Source: CAD feature listing. Evaluate the final solid. Frame: model axes, mm. A direction names the side the tool comes from. Round coordinates to 2 decimals unless told otherwise and drop trailing zeros. Loops run counter-clockwise (first coordinate to the right, second up) from the corner with the lowest first, then second, coordinate; pieces in that order, holes last.
(1) Material intervals for probe 1 along Z at (x, y) = (-35.5, 1.35); probe 2 along X at (y, z) = (0.1, -15); probe 3 along Z at (x, y) = (-11.5, 1.3), sorted ascending.
(2) Section A-A, the plane x = 0. Return the cut outline in (y, z) (3 decimals), plus the area to 3 significant figures.
(3) Section D-D, the plane y = 1.5. Count the separate pieces of the cut face and the enclosed holes in it, plus the area to 3 significant figures.
(4) Section C-C, the plane x = -12.5. Return the cut outline in (y, z), plus the area to 3 significant figures.
(5) Set-up query: faces 1 (the flat face through (1, 0, 1)), 2 (the cylindrical face through (-22.106, 0.986, -21.846)). Return all of +Z, -Z, +X, -X, +Y, -Y with unobstructed straight access to the full face (end or side cutting, diameter ignored); none if empty.
(6) Section B-B, the plane z = 0. Return the cut outline in (x, y), plus the area to 3 significant figures.
(7) First-contact query: pin 1 Ø5 at (x, z) = (35.75, 20.64) entering from +Y; pin 2 Ø1.9 at (x, z) = (0, -41.275) entering from -Y. Flat tips, straight axial feed; report the tip coordinate or a pass-through.
Autodesk Inventor part; units mm, degrees
ref_plane "YZ Plane" through (0, 0, 0) normal (1, 0, 0) x (0, 1, 0)
ref_plane "XZ Plane" through (0, 0, 0) normal (0, 1, 0) x (-1, 0, 0)
ref_plane "XY Plane" through (0, 0, 0) normal (0, 0, 1) x (1, 0, 0)
sketch "Sketch1" plane through (0, 0, 0) normal (0, 1, 0) x (-1, 0, 0)
  circle A0 centre (0, 0) radius 44.45
  circle A1 centre (0, -41.275) radius 1.6
  circle A2 centre (35.7452, -20.6375) radius 1.6
  circle A3 centre (-35.7452, -20.6375) radius 1.6
  circle A4 centre (0, 41.275) radius 1.6
  circle A5 centre (35.7452, 20.6375) radius 1.6
  circle A6 centre (-35.7452, 20.6375) radius 1.6
  arc A7 (28.0281, -10.5398) -> (10.5398, -28.0281) centre (12.7279, -12.7279) ccw
  arc A8 (10.5398, -28.0281) -> (28.0281, -10.5398) centre (6.4322, -6.4322) ccw
extrude "Extrusion1" add sketch "Sketch1" along normal blind 2
properties part number "Dremel_Jig_Internall"
Output values:
1. probe 1: z = -26.75 to -22.22, -19.06 to 19.06, 22.22 to 26.75
1. probe 2: x = -41.84 to -26.68, 2.56 to 41.84
1. probe 3: z = -42.94 to -27.82, 2.68 to 42.94
2. outline: (0, -44.45) - (2, -44.45) - (2, -42.875) - (0, -42.875) - close; (0, -39.675) - (2, -39.675) - (2, -21.496) - (0, -21.496) - close; (0, -3.96) - (2, -3.96) - (2, 39.675) - (0, 39.675) - close; (0, 42.875) - (2, 42.875) - (2, 44.45) - (0, 44.45) - close
2. area: 130 mm2
3. separate pieces: 1
3. enclosed holes: 7
3. area: 5,450 mm2
4. outline: (0, -42.66) - (2, -42.66) - (2, -27.56) - (0, -27.56) - close; (0, 2.73) - (2, 2.73) - (2, 42.66) - (0, 42.66) - close
4. area: 110 mm2
5. face 1: +Z, -Z, +X, -X, -Y
5. face 2: +Y, -Y
6. outline: (-44.45, 0) - (-21.5, 0) - (-21.5, 2) - (-44.45, 2) - close; (-3.96, 0) - (44.45, 0) - (44.45, 2) - (-3.96, 2) - close
6. area: 143 mm2
7. pin 1: stops at y = 2
7. pin 2: passes through
